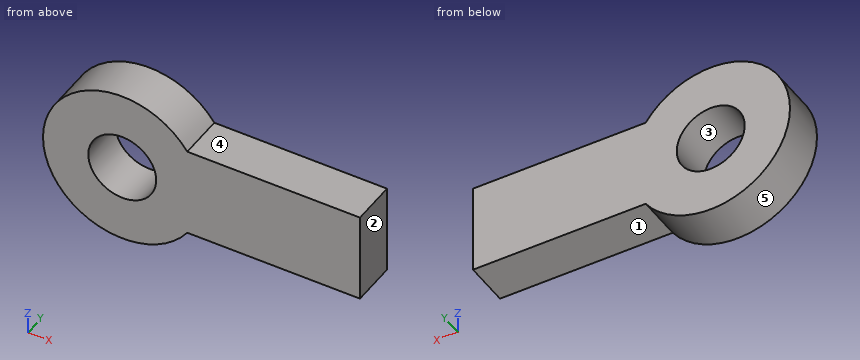
```python
from build123d import *

# Parameters (mm, degrees)
SZKIC1_R                    = 1.5
DODANIE_WYCI_GNI_CIE1_DEPTH = 2


with BuildPart() as part:
    # Szkic1 → Dodanie-wyciągnięcie1 (new body)
    with BuildSketch(Plane(origin=(0, 0, 0), x_dir=(1, 0, 0), z_dir=(0, 1, 0))):
        with BuildLine():
            Line((3.5, 2), (10.5, 2))
            Line((10.5, 2), (10.5, -2))
            Line((10.5, -2), (3.5, -2))
            Line((3.5, -2), (2.872281323, -2))
            ThreePointArc((2.872281323, -2), (-3.5, 0), (2.872281323, 2))
            Line((2.872281323, 2), (3.5, 2))
        make_face()
        with Locations(Location((0, 0, 0), (0, 0, 270))):
            Circle(SZKIC1_R, mode=Mode.SUBTRACT)
    extrude(amount=DODANIE_WYCI_GNI_CIE1_DEPTH)


solid = part.part
```
Here's how the part is built. I have some questions about the finished solid (model axes, mm). Face numbers are marked on the shaded views. A direction names the side the tool comes from. Give positions to 0.01 mm unless a question says otherwise; leave off trailing zeros. Order: outer loops, then holes, each group sorted by start corner. A loop starts at its lowest first (then second) coordinate and runs counter-clockwise, first axis right, second up. Notation, with made-up numbers: M -7,-31.75 L 13,-31.75 A16 cw 13,-6.75 Z; hole C 79,-3 d2. An arc over 180 degrees is marked long. Use a Markdown table: item, result. Add a question column.
1. Suppose I cut it at B-B (x = 0). List the corners of the cut face in (y, z) for me, and give its area (3 significant figures).
2. Suppose I cut it at D-D (x = 6.75). List the corners of the cut face in (y, z) for me.
3. I need wall thicknesses on probe 1 along X at (y, z) = (1.5, 0); probe 2 along Z at (x, y) = (3, 0.6); probe 3 along X at (y, z) = (0.9, -1.25). Which ranges of each line are inside material? Lowest first, please. Write a range as from..to.
4. If we mould it in two halves opening along X, with no side actions, what happens to the marked faces 3, 4 and 5? For each: +X half, -X half, draft (parallel to the pull), parting line (faces both ways), or undercut.
5. Suppose I cut it at C-C (y = 1.15). List the corners of the cut face in (x, z) for me.
6. On a 3-axis mill with a long thin cutter (end or side, diameter ignored), from which of +Z, -Z, +X, -X, +Y, -Y can I reach the whole of each face in a straight line? I mean the marked faces 1 and 2. Say none if no direction works.
7. Suppose I cut it at A-A (z = 0). List the corners of the cut face in (x, y) for me, and give its area (3 significant figures).
8. For pin 1 Ø1 at (x, y) = (8.5, 1) entering from +Z, with a flat end and sliding along its axis, tell me the tip position at first contact or that it passes through.
Results list:
| question | item | result |
|---|---|---|
| 1 | outline | M 0,-3.5 L 2,-3.5 L 2,-1.5 L 0,-1.5 Z; M 0,1.5 L 2,1.5 L 2,3.5 L 0,3.5 Z |
| 1 | area | 8.00 mm² |
| 2 | outline | M 0,-2 L 2,-2 L 2,2 L 0,2 Z |
| 3 | probe 1 | x = -3.5..-1.5, 1.5..10.5 |
| 3 | probe 2 | z = -2..2 |
| 3 | probe 3 | x = -3.27..-0.83, 0.83..10.5 |
| 4 | face 3 | undercut |
| 4 | face 4 | draft |
| 4 | face 5 | parting line |
| 5 | outline | M 2.87,-2 L 10.5,-2 L 10.5,2 L 2.87,2 A3.5 ccw long Z; hole C 0,0 d3 |
| 6 | face 1 | -Z, +X, +Y, -Y |
| 6 | face 2 | +Z, -Z, +X, +Y, -Y |
| 7 | outline | M -3.5,0 L -1.5,0 L -1.5,2 L -3.5,2 Z; M 1.5,0 L 10.5,0 L 10.5,2 L 1.5,2 Z |
| 7 | area | 22.0 mm² |
| 8 | pin 1 | stops at z = 2 |
